Can you work these out from the model? Positions are in its coordinate system, mm. Face numbers are marked on the shaded views. Give positions to 0.01 mm unless a question says otherwise; leave off trailing zeros. Loops run counter-clockwise (first coordinate to the right, second up) from the corner with the lowest first, then second, coordinate; pieces in that order, holes last. Notation, with made-up numbers: (73.25, 17) - (125.25, 17) arc R23 ccw to (125.25, 42) - close; hole circle Ø8 at (-25, -2.75). An arc over 180 degrees is marked (long way). Answer in a Markdown table with one row per item.
from build123d import *

# Parameters (mm, degrees)
SKETCH_1_R                      = 12.55
EXTRUDE_1_DEPTH                 = 9
CUT_EXTRUDE_1_REACH             = 21.9
SKETCH_2_R                      = 3.2
CUT_EXTRUDE_2_REACH             = 21.9
SKETCH_3_R                      = 1
CUT_EXTRUDE_2_DIRECTION_2_REACH = 21.9
CUT_EXTRUDE_3_DEPTH             = 21
CUT_EXTRUDE_3_DEPTH_BACK        = 19
SKETCH_4_R                      = 1


with BuildPart() as part:
    # 草图1 → 凸台-拉伸1 (new body)
    with BuildSketch(Plane(origin=(0, 0, 0), x_dir=(0, 0, -1), z_dir=(1, 0, 0))):
        Circle(SKETCH_1_R)
    extrude(amount=EXTRUDE_1_DEPTH)

    # 草图2 → 切除-拉伸1 (cut, up to next)
    with BuildSketch(Plane.ZY, mode=Mode.PRIVATE) as cut_extrude_1_sk1:
        Circle(SKETCH_2_R)
    cut_extrude_1_tool1 = extrude(cut_extrude_1_sk1.sketch, amount=-CUT_EXTRUDE_1_REACH, mode=Mode.PRIVATE) & part.part
    add(cut_extrude_1_tool1.solids().sort_by_distance((0, 0, 0))[0], mode=Mode.SUBTRACT)

    # 草图3 → 切除-拉伸2 (cut, up to next)
    with BuildSketch(Plane(origin=(0, 0, 0), x_dir=(1, 0, 0), z_dir=(0, 1, 0)), mode=Mode.PRIVATE) as cut_extrude_2_sk1:
        with Locations(Location((3, 0, 0), (0, 0, 270))):
            Circle(SKETCH_3_R)
    cut_extrude_2_tool1 = extrude(cut_extrude_2_sk1.sketch, amount=-CUT_EXTRUDE_2_REACH, mode=Mode.PRIVATE) & part.part
    add(cut_extrude_2_tool1.solids().sort_by_distance((3, 0, 0))[0], mode=Mode.SUBTRACT)

    # 草图3 → 切除-拉伸2 direction 2 (cut, up to next)
    with BuildSketch(Plane(origin=(0, 0, 0), x_dir=(1, 0, 0), z_dir=(0, 1, 0)), mode=Mode.PRIVATE) as cut_extrude_2_direction_2_sk1:
        with Locations(Location((3, 0, 0), (0, 0, 270))):
            Circle(SKETCH_3_R)
    cut_extrude_2_direction_2_tool1 = extrude(cut_extrude_2_direction_2_sk1.sketch, amount=CUT_EXTRUDE_2_DIRECTION_2_REACH, mode=Mode.PRIVATE) & part.part
    add(cut_extrude_2_direction_2_tool1.solids().sort_by_distance((3, 0, 0))[0], mode=Mode.SUBTRACT)

    # 草图4 → 切除-拉伸3 (cut, two sides: drawn at the far end of the back side and taken through both)
    with BuildSketch(Plane.XY.offset(-CUT_EXTRUDE_3_DEPTH_BACK)):
        with Locations(Location((6, 0, 0), (0, 0, 180))):
            Circle(SKETCH_4_R)
    extrude(amount=CUT_EXTRUDE_3_DEPTH + CUT_EXTRUDE_3_DEPTH_BACK, mode=Mode.SUBTRACT)


solid = part.part
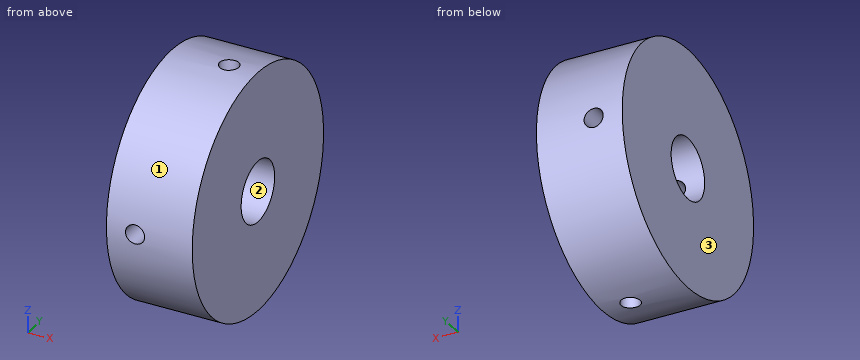
Q1. Imagine slicing it at D-D, the plane y = 8. Write out the boundary of the cut face in (x, z).
Checked values:
| item | result |
|---|---|
| outline | (0, -9.67) - (9, -9.67) - (9, 9.67) - (0, 9.67) - close; hole circle Ø2 at (3, 0) |
Q2. Imagine slicing it at B-B, the plane y = 0. Write out the boundary of the cut face in (x, z), and give its area (3 significant figures).
Checked values:
| item | result |
|---|---|
| outline | (0, -12.55) - (5, -12.55) - (5, -3.2) - (0, -3.2) - close; (0, 3.2) - (5, 3.2) - (5, 12.55) - (0, 12.55) - close; (7, -12.55) - (9, -12.55) - (9, -3.2) - (7, -3.2) - close; (7, 3.2) - (9, 3.2) - (9, 12.55) - (7, 12.55) - close |
| area | 131 mm² |
Q3. If we mould it in two halves opening along Y, with no side actions, what happens to the marked faces 1, 2 and 3? For each: released by +Y, released by -Y, zero draft, split by the parting line, or undercut.
Checked values:
| item | result |
|---|---|
| face 1 | split by the parting line |
| face 2 | undercut |
| face 3 | zero draft |
Q4. For pin 1 (2.5 mm diameter, centred on x = 6, y = 0, fed in from +Z); pin 2 (2 mm diameter, centred on x = 7, y = 1.5, fed in from -Z); pin 3 (1.5 mm diameter, centred on x = 4.5, y = 9.5, fed in from -Z); pin 4 (1.8 mm diameter, centred on x = 3, z = 0, fed in from -Y), each with a flat end and sliding along its axis, tell me the tip position at first contact or that it passes through.
Checked values:
| item | result |
|---|---|
| pin 1 | stops at z = 12.55 |
| pin 2 | stops at z = -12.54 |
| pin 3 | stops at z = -9 |
| pin 4 | passes through |
Q5. If I drill on line 1 (Y direction, x = 5, z = 0); line 2 (Y direction, x = 6, z = 6); line 3 (Z direction, x = 4, y = -2.5), over which ranges is the centre line in solid material (lowest first)? Write a range as [from, to].
Checked values:
| item | result |
|---|---|
| line 1 | y = [-12.55, -3.2], [3.2, 12.55] |
| line 2 | y = [-11.02, -1], [1, 11.02] |
| line 3 | z = [-12.3, -2], [2, 12.3] |
Q6. Imagine slicing it at A-A, the plane z = 0. Write out the boundary of the cut face in (x, y).
Checked values:
| item | result |
|---|---|
| outline | (0, -12.55) - (2, -12.55) - (2, -3.2) - (0, -3.2) - close; (0, 3.2) - (2, 3.2) - (2, 12.55) - (0, 12.55) - close; (4, -12.55) - (9, -12.55) - (9, -3.2) - (4, -3.2) - close; (4, 3.2) - (9, 3.2) - (9, 12.55) - (4, 12.55) - close |
Q7. Imagine slicing it at C-C, the plane x = 6. Write out the boundary of the cut face in (y, z), and give its area (3 significant figures).
Checked values:
| item | result |
|---|---|
| outline | (-1, -12.51) - (-1, -3.04) arc R3.2 cw to (-1, 3.04) - (-1, 12.51) arc R12.55 ccw to start; (1, -12.51) arc R12.55 ccw to (1, 12.51) - (1, 3.04) arc R3.2 cw to (1, -3.04) - close |
| area | 425 mm² |
